from build123d import *

# Parameters (mm, degrees)
MAIN_EXTRUSION_DEPTH             = 350
MOUNTING_HOLE_MASTER_D           = 3.5
MOUNTING_HOLE_MASTER_DEPTH       = 9.921567416
MOUNTING_HOLE_MASTER_CBORE_D     = 6
MOUNTING_HOLE_MASTER_CBORE_DEPTH = 4.5
MOUNTING_HOLES_PATTERN_COUNT     = 14
MOUNTING_HOLES_PATTERN_PITCH     = 25
RAIL_TOP_CHAMFER_SIZE            = 0.5
RAIL_BOTTOM_CHAMFER_SIZE         = 1


with BuildPart() as part:
    # MainProfile → Main Extrusion (new body)
    with BuildSketch(Plane.XY):
        Polygon((0, 0), (0, 3.585786438), (0.707106781, 4.292893219), (1.707106781, 4.292893219), (1.707106781, 5.292893219), (0.707106781, 5.292893219), (0, 6), (0, 8), (12, 8), (12, 6), (11.292893219, 5.292893219), (10.292893219, 5.292893219), (10.292893219, 4.292893219), (11.292893219, 4.292893219), (12, 3.585786438), (12, 0), align=None)
    extrude(amount=MAIN_EXTRUSION_DEPTH)

    # Mounting Hole Master
    with Locations(Plane(origin=(0, 8, 0), x_dir=(1, 0, 0), z_dir=(0, 1, 0))):
        with Locations((6, -10)):
            mounting_hole_master = CounterBoreHole(MOUNTING_HOLE_MASTER_D / 2, MOUNTING_HOLE_MASTER_CBORE_D / 2, MOUNTING_HOLE_MASTER_CBORE_DEPTH, depth=MOUNTING_HOLE_MASTER_DEPTH)

    # Mounting Holes Pattern: Mounting Hole Master ×14
    with Locations(*[(0, 0, i * MOUNTING_HOLES_PATTERN_PITCH) for i in range(1, MOUNTING_HOLES_PATTERN_COUNT)]):
        add(mounting_hole_master, mode=Mode.SUBTRACT)

    # Rail Top Chamfer
    rail_top_chamfer_edges = [part.edges().sort_by_distance(p)[0] for p in [
        (12, 8, 175),
        (0, 8, 175),
    ]]
    chamfer(rail_top_chamfer_edges, length=RAIL_TOP_CHAMFER_SIZE)

    # Rail Bottom Chamfer
    rail_bottom_chamfer_edges = [part.edges().sort_by_distance(p)[0] for p in [
        (0, 0, 175),
        (12, 0, 175),
    ]]
    chamfer(rail_bottom_chamfer_edges, length=RAIL_BOTTOM_CHAMFER_SIZE)


solid = part.part
Can you work these out from the model? Positions are in its coordinate system, mm. Coordinates: 2 decimals unless noted, no trailing zeros. Write each loop counter-clockwise with the first axis right and the second up, starting at its lowest first coordinate (ties: lowest second). Pieces come first, ordered by that corner, then holes. Notation, with made-up numbers: (-18, 88) - (37, 88) arc R16 ccw to (37, 111) - close; hole circle Ø3 at (9.25, -13). An arc over 180 degrees is marked (long way). Return JSON: item names as keys, results as strings. Group by question number.
Item 1: I'm going to push a flat-ended pin straight in: pin 1 Ø4 at (x, z) = (6, 335) entering from +Y. Where does the tip first touch, or does it pass through?
Item 2: We'd pull the mould along Z, two halves only. Please class faces 1 (the face through (8, 3.5, 285)), 2 (the face through (6, 0, 173)), 3 (the face through (6, 4, 0)), 4 (the face through (6, 6, 232)): pulls with the +Z half, pulls with the -Z half, needs draft (parallel to the pull), parting line crosses it, or undercut.
Item 3: If we section it at A-A (z = 277): Write out the boundary of the cut face in (x, y), then the cut area to 3 significant figures.
Item 4: Please list where these lines run through material, in increasing order: probe 1 along Y at (x, z) = (10.5, 30); probe 2 along X at (y, z) = (4.85, 60); probe 3 along X at (y, z) = (2.05, 135).
Return value:
{
 "1": {"pin 1": "stops at y = 3.5"},
 "2": {"face 1": "undercut", "face 2": "needs draft", "face 3": "pulls with the -Z half", "face 4": "undercut"},
 "3": {"outline": "(0, 1) - (1, 0) - (11, 0) - (12, 1) - (12, 3.59) - (11.29, 4.29) - (10.29, 4.29) - (10.29, 5.29) - (11.29, 5.29) - (12, 6) - (12, 7.5) - (11.5, 8) - (0.5, 8) - (0, 7.5) - (0, 6) - (0.71, 5.29) - (1.71, 5.29) - (1.71, 4.29) - (0.71, 4.29) - (0, 3.59) - close", "area": "90.3 mm^2"},
 "4": {"probe 1": "y = 0 to 4.29, 5.29 to 8", "probe 2": "x = 1.71 to 3, 9 to 10.29", "probe 3": "x = 0 to 4.25, 7.75 to 12"}
}
